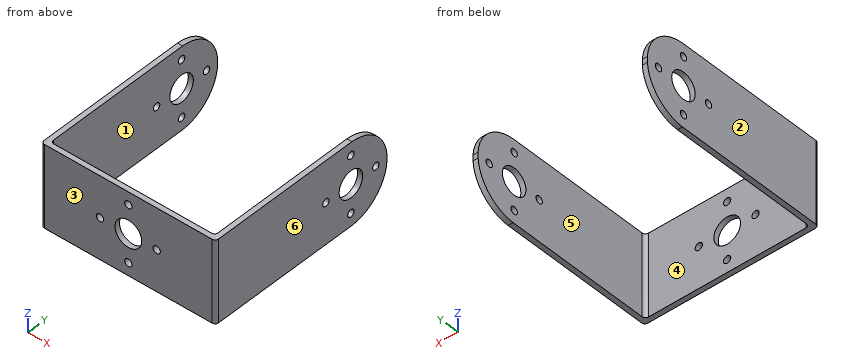
from build123d import *

# Parameters (mm, degrees)
BOSS_EXTRUDE1_DEPTH    = 24.61
CUT_EXTRUDE5_START     = -1.52
CUT_EXTRUDE5_OUTLINE_R = 4
CUT_EXTRUDE5_DEPTH     = 1.52
SKETCH4_R              = 1.09
CUT_EXTRUDE6_DEPTH     = 100
CIRPATTERN1_COUNT      = 4
SKETCH5_R              = 4
CUT_EXTRUDE7_DEPTH     = 50
SKETCH6_R              = 1.09
CUT_EXTRUDE8_DEPTH     = 50
CIRPATTERN2_COUNT      = 4
FILLET1_R              = 1


# Read off the part's stored shape, not the designer's step: Cut-Extrude5
with BuildPart() as part:
    # Sketch1 → Boss-Extrude1 (new body)
    with BuildSketch(Plane.XY):
        Polygon((-26.125, 58.34), (-26.125, 0), (26.125, 0), (26.125, 58.34), (24.605, 58.34), (24.605, 1.52), (-24.605, 1.52), (-24.605, 58.34), align=None)
    extrude(amount=BOSS_EXTRUDE1_DEPTH)

    # Cut-Extrude5 outline → Cut-Extrude5 (cut)
    with BuildSketch(Plane.ZY.offset(26.125).offset(CUT_EXTRUDE5_START)):
        with BuildLine():
            ThreePointArc((0, 46.410820467), (3.42252503, 54.582777623), (11.446105362, 58.34))
            Line((11.446105362, 58.34), (0, 58.34))
            Line((0, 58.34), (0, 46.410820467))
        make_face()
        with BuildLine():
            Line((24.61, 58.34), (13.163894638, 58.34))
            ThreePointArc((13.163894638, 58.34), (21.18747497, 54.582777623), (24.61, 46.410820467))
            Line((24.61, 46.410820467), (24.61, 58.34))
        make_face()
        with Locations((12.305, 46.06)):
            Circle(CUT_EXTRUDE5_OUTLINE_R)
    cut_extrude5 = extrude(amount=CUT_EXTRUDE5_DEPTH, mode=Mode.SUBTRACT)

    # Mirror1: Cut-Extrude5 across plane
    add(cut_extrude5.mirror(Plane(origin=(0, 0, 0), x_dir=(0, 0, 1), z_dir=(1, 0, 0))), mode=Mode.SUBTRACT)

    # Sketch4 → Cut-Extrude6 (cut)
    with BuildSketch(Plane.ZY.offset(26.125)):
        with Locations(Location((12.305, 54.56, 0), (0, 0, 270))):
            Circle(SKETCH4_R)
    cut_extrude6 = extrude(amount=-CUT_EXTRUDE6_DEPTH, mode=Mode.SUBTRACT)

    # CirPattern1: Cut-Extrude6 ×4 about axis
    cirpattern1_axis = Axis((0, 46.06, 12.305), (1, 0, 0))
    for i in range(1, CIRPATTERN1_COUNT):
        add(cut_extrude6.rotate(cirpattern1_axis, i * 360 / CIRPATTERN1_COUNT), mode=Mode.SUBTRACT)

    # Sketch5 → Cut-Extrude7 (cut, symmetric)
    with BuildSketch(Plane(origin=(0, 1.52, 0), x_dir=(1, 0, 0), z_dir=(0, 1, 0))):
        with Locations(Location((0, -12.305, 0), (0, 0, 270))):
            Circle(SKETCH5_R)
    extrude(amount=CUT_EXTRUDE7_DEPTH, both=True, mode=Mode.SUBTRACT)

    # Sketch6 → Cut-Extrude8 (cut, symmetric)
    with BuildSketch(Plane(origin=(0, 1.52, 0), x_dir=(1, 0, 0), z_dir=(0, 1, 0))):
        with Locations(Location((0, -3.805, 0), (0, 0, 270))):
            Circle(SKETCH6_R)
    cut_extrude8 = extrude(amount=CUT_EXTRUDE8_DEPTH, both=True, mode=Mode.SUBTRACT)

    # CirPattern2: Cut-Extrude8 ×4 about axis
    cirpattern2_axis = Axis((0, 0, 12.305), (0, 1, 0))
    for i in range(1, CIRPATTERN2_COUNT):
        add(cut_extrude8.rotate(cirpattern2_axis, i * 360 / CIRPATTERN2_COUNT), mode=Mode.SUBTRACT)

    # Fillet1
    fillet1_edges = [part.edges().sort_by_distance(p)[0] for p in [
        (-24.605, 1.52, 12.305),
        (24.605, 1.52, 12.305),
        (26.125, 0, 12.305),
        (-26.125, 0, 12.305),
    ]]
    fillet(fillet1_edges, radius=FILLET1_R)


solid = part.part
Work out the finished part from the listing and answer in its coordinate system (mm). Face numbers are marked on the shaded views. A direction names the side the tool comes from. Round coordinates to 2 decimals unless told otherwise and drop trailing zeros. Order: outer loops, then holes, each group sorted by start corner. A loop starts at its lowest first (then second) coordinate and runs counter-clockwise, first axis right, second up. Notation, with made-up numbers: M 58.5,-8.75 L 104.5,-8.75 A7 cw 104.5,1.25 Z; hole C 22.25,7 d9. An arc over 180 degrees is marked long. Put each result on its own line as item: value. Start each with the question number.
Q1. For a pull along X with two mould halves and no side action, classify the marked faces 1, 2, 3 and 4 as pulls with the +X half, pulls with the -X half, needs draft (parallel to the pull), parting line crosses it, or undercut.
Q2. A tool of negligible diameter and unlimited length cuts with its end or side. For the marked faces 5 and 6, from which of +Z, -Z, +X, -X, +Y, -Y can it reach the whole face along a straight path? Write none if from no direction.
Q3. Section C-C, the plane x = 0 is taken. Write down the section's boundary in (y, z) (3 decimals).
Q4. Section B-B, the plane x = -8.5 is taken. Write down the section's boundary in (y, z) (3 decimals).
Q5. Straight lines are drawn through the part: L1, parallel to X at y = 51, z = 21.5 (3 decimals); L2, parallel to Y at x = -19, z = 12.75; L3, parallel to X at y = 2, z = 23 (3 decimals). For each, find the intervals that lie inside material, in ascending order. Write a range as [from, to].
Q6. Section D-D, the plane y = 28.5 is taken. Write down the section's boundary in (x, z) (3 decimals).
Q7. Flat-ended cylindrical pins translate along their axes: pin 1 (5 mm diameter, centred on x = 7, z = 20.5, fed in from +Y); pin 2 (2 mm diameter, centred on x = -8.5, z = 12.305, fed in from -Y). Find the tip coordinate at first contact, or state that the pin passes through.
Q8. Section A-A, the plane y = 37.56 is taken. Write down the section's boundary in (x, z) (3 decimals).
Findings below:
1. face 1: undercut
1. face 2: pulls with the -X half
1. face 3: needs draft
1. face 4: undercut
2. face 5: +Z, -Z, +Y
2. face 6: +Z, -Z, +X, +Y, -Y
3. outline: M 0,0 L 1.52,0 L 1.52,2.715 L 0,2.715 Z; M 0,4.895 L 1.52,4.895 L 1.52,8.305 L 0,8.305 Z; M 0,16.305 L 1.52,16.305 L 1.52,19.715 L 0,19.715 Z; M 0,21.895 L 1.52,21.895 L 1.52,24.61 L 0,24.61 Z
4. outline: M 0,0 L 1.52,0 L 1.52,11.215 L 0,11.215 Z; M 0,13.395 L 1.52,13.395 L 1.52,24.61 L 0,24.61 Z
5. L1: x = [-26.125, -24.605], [24.605, 26.125]
5. L2: y = [0, 1.52]
5. L3: x = [-26.125, -24.459], [24.459, 26.125]
6. outline: M -26.125,0 L -24.605,0 L -24.605,24.61 L -26.125,24.61 Z; M 24.605,0 L 26.125,0 L 26.125,24.61 L 24.605,24.61 Z
7. pin 1: stops at y = 1.52
7. pin 2: passes through
8. outline: M -26.125,0 L -24.605,0 L -24.605,11.215 L -26.125,11.215 Z; M -26.125,13.395 L -24.605,13.395 L -24.605,24.61 L -26.125,24.61 Z; M 24.605,0 L 26.125,0 L 26.125,11.215 L 24.605,11.215 Z; M 24.605,13.395 L 26.125,13.395 L 26.125,24.61 L 24.605,24.61 Z
